```python
from build123d import *

# Parameters (mm, degrees)
UPPER_DEPTH = 1.5
SKETCH2_R   = 2.159
LOWER_DEPTH = 1.5


with BuildPart() as part:
    # Sketch1 → Upper (new body)
    with BuildSketch(Plane.XY):
        Polygon((-212.5, 0), (212.5, 0), (266.41785, -250), (-266.41785, -250), align=None)
    extrude(amount=UPPER_DEPTH)

    # Sketch2 → Lower (add)
    with BuildSketch(Plane(origin=(0, -125.523597244, -124.998903379), x_dir=(1, 0, 0), z_dir=(0, 0.70858619, 0.70562427))):
        Polygon((-187.8166, -793.662967608), (187.8166, -793.662967608), (267.44325, -518.175167608), (292.1, -383.391867608), (266.41785, -176.406067608), (-266.41785, -176.406067608), (-292.1, -383.391867608), (-267.44325, -518.175167608), align=None)
        Polygon((-290.093306858, -367.218884221), (-268.844696442, -195.965284898), (-282.847719378, -194.227833655), (-304.096329794, -365.481432978), align=None)
        with Locations((-286.940102201, -280.648769571)):
            Circle(SKETCH2_R, mode=Mode.SUBTRACT)
        Polygon((282.847719378, -194.227833655), (268.844696442, -195.965284898), (290.093306858, -367.218884221), (304.096329794, -365.481432978), align=None)
        with Locations((286.940102201, -280.648769571)):
            Circle(SKETCH2_R, mode=Mode.SUBTRACT)
    extrude(amount=LOWER_DEPTH)


solid = part.part
```
The model under review builds one solid part; all positions refer to its coordinate system, in mm. A direction names the side the tool comes from. Round coordinates to 2 decimals unless told otherwise and drop trailing zeros. Loops run counter-clockwise (first coordinate to the right, second up) from the corner with the lowest first, then second, coordinate; pieces in that order, holes last.
Item 1: For line 1 (Z direction, x = 91, y = -67); line 2 (Z direction, x = -260, y = -411.5); line 3 (Y direction, x = -9.5, z = 307), list the stretches that pass through material, from the lowest coordinate up.
Determined:
line 1: z = 0 to 1.5
line 2: z = 162.18 to 164.3
line 3: y = -555.72 to -553.6
Item 2: Clearance check with flat-ended pins moving along their axes: pin 1 Ø12 at (x, y) = (-152.5, -517) entering from +Z; pin 2 Ø3 at (x, y) = (-141.5, -281) entering from +Z; pin 3 Ø4 at (x, y) = (-36, -318.5) entering from -Z. State where each tip first meets the part, or that it passes through.
Determined:
pin 1: stops at z = 276.27
pin 2: stops at z = 34.76
pin 3: stops at z = 66.78
Item 3: Take a section at A-A (x = -127). Write out the cut boundary in (y, z), then the cut area to 3 significant figures.
Determined:
outline: (-685.55, 437.38) - (-250, 0) - (0, 0) - (0, 1.5) - (-249.38, 1.5) - (-684.49, 438.44) - close
area: 1,300 mm2
Item 4: Take a section at D-D (x = -252). Write out the cut boundary in (y, z), then the cut area to 3 significant figures.
Determined:
outline: (-528.86, 280.03) - (-250, 0) - (-183.15, 0) - (-183.15, 1.5) - (-249.38, 1.5) - (-527.8, 281.09) - close
area: 692 mm2
Item 5: Take a section at B-B (y = -412). Write out the cut boundary in (x, z), then the cut area to 3 significant figures.
Determined:
outline: (-287.97, 162.68) - (287.97, 162.68) - (287.69, 164.81) - (-287.69, 164.81) - close
area: 1,220 mm2
Item 6: Take a section at C-C (z = 120.5). Write out the cut boundary in (x, y).
Determined:
outline: (-301.74, -370) - (301.74, -370) - (301.55, -367.88) - (-301.55, -367.88) - close
Item 7: For faces 1 (the face through (227.073, -589.193, 341.665)), 2 (the face through (4, -123, 1.5)), list the 3-axis set-ups (+Z, -Z, +X, -X, +Y, -Y) from which the entire face can be reached by the end or side of a thin tool; tool diameter is ignored.
Determined:
face 1: +Z, +X, -Y
face 2: +Z, +X, -X, +Y
